Verification items for the finished model (mm, model axes). A direction names the side the tool comes from. Give positions to 0.01 mm unless a question says otherwise; leave off trailing zeros. Order: outer loops, then holes, each group sorted by start corner. A loop starts at its lowest first (then second) coordinate and runs counter-clockwise, first axis right, second up. Notation, with made-up numbers: (70, 63.5) - (113, 63.5) arc R20 cw to (113, 82.5) - close; hole circle Ø1 at (-15.5, 3). An arc over 180 degrees is marked (long way). Answer as a JSON object with one key per item and string values. Group by question number.
(1) Mould release check, pull along Z, two halves, no side actions. Record for faces 6 (the face through (2.465, -7.413, -11.197)), 7 (the face through (2.465, 7.345, -11.241)), 8 (the face through (-3, 0, 10)), 9 (the face through (2.46, 12.85, -3.89)): +Z half, -Z half, draft (parallel to the pull), parting line (faces both ways), or undercut.
(2) Thickness scan on line 1 (Y direction, x = 3.55, z = 0); line 2 (Y direction, x = 4, z = 12.5); line 3 (Y direction, x = -4.25, z = 0). Record the ranges inside material, lowest first.
(3) Section check B-B (y = -9.25). Record the boundary of the cut face in (x, z), then the cut area to 3 significant figures.
(4) Section check A-A (x = -4.5). Record the boundary of the cut face in (y, z), then the cut area to 3 significant figures.
(5) Depth check by flat-ended pin: pin 1 Ø0.9 at (y, z) = (0.5, 5.5) entering from -X; pin 2 Ø1 at (x, y) = (1.5, 9) entering from -Z; pin 3 Ø6 at (x, z) = (-4.5, 11.5) entering from -Y. Enter the tip coordinate at first touch or a pass-through.
(6) Access from +Z, -Z, +X, -X, +Y, -Y to the whole of each face (thin tool, end or side, straight path). Record for faces 1 (the face through (2.46, -0.71, 12.23)), 2 (the face through (2.465, -12.842, 3.814)), 3 (the face through (2.46, 13.4, -0.82)), 4 (the face through (2.465, -10.747, 8.051)), 5 (the face through (2.465, -4.631, -12.605)).
```python
from build123d import *

# Parameters (mm, degrees)
BASPROSKE_W         = 5
BASPROSKE_H         = 14.5
TOOTHCUT_DEPTH      = 22.106870919
TEETHCUTS_COUNT     = 27
TEETHCUTS_ANGLE     = 346.666666667
BORSKE_R            = 1.5
BORE_DEPTH          = 50.0000508
SKETCH2_R           = 10
BOSS_EXTRUDE1_DEPTH = 7
CUT_EXTRUDE3_START  = -7
SKETCH3_R           = 1.5
CUT_EXTRUDE3_DEPTH  = 7


with BuildPart() as part:
    # BasProSke → Base-Revolve (revolve)
    with BuildSketch(Plane(origin=(0, 0, 0), x_dir=(1, 0, 0), z_dir=(0, 1, 0)), mode=Mode.PRIVATE) as base_revolve_sk:
        with Locations((2.5, 7.25)):
            Rectangle(BASPROSKE_W, BASPROSKE_H)
    revolve(base_revolve_sk.sketch.rotate(Axis((-10, 0, 0), (1, 0, 0)), 180), axis=Axis((-10, 0, 0), (1, 0, 0)))

    # TooCutSke → ToothCut (cut, through all)
    with BuildSketch(Plane(origin=(0, 0, 0), x_dir=(0, 0, -1), z_dir=(1, 0, 0))):
        with BuildLine():
            ThreePointArc((0.474054864, 12.239823242), (0, 12.249), (-0.474054864, 12.239823242))
            ThreePointArc((-0.474054864, 12.239823242), (-0.820231692, 13.40120918), (-1.416685779, 14.456149092))
            ThreePointArc((-1.416685779, 14.456149092), (0, 14.5254), (1.416685779, 14.456149092))
            ThreePointArc((1.416685779, 14.456149092), (0.820231692, 13.40120918), (0.474054864, 12.239823242))
        make_face()
    toothcut = extrude(amount=TOOTHCUT_DEPTH, mode=Mode.SUBTRACT)

    # TeethCuts: ToothCut ×27 about axis
    teethcuts_axis = Axis((-10, 0, 0), (1, 0, 0))
    for i in range(1, TEETHCUTS_COUNT):
        add(toothcut.rotate(teethcuts_axis, i * TEETHCUTS_ANGLE / (TEETHCUTS_COUNT - 1)), mode=Mode.SUBTRACT)

    # BorSke → Bore (cut, symmetric)
    with BuildSketch(Plane(origin=(0, 0, 0), x_dir=(0, 0, -1), z_dir=(1, 0, 0))):
        with Locations(Location((0, 0, 0), (0, 0, 180))):
            Circle(BORSKE_R)
    extrude(amount=BORE_DEPTH, both=True, mode=Mode.SUBTRACT)

    # Sketch2 → Boss-Extrude1 (add)
    with BuildSketch(Plane.ZY):
        with Locations(Location((0, 0, 0), (0, 0, 180))):
            Circle(SKETCH2_R)
    extrude(amount=BOSS_EXTRUDE1_DEPTH)

    # Sketch3 → Cut-Extrude3 (cut)
    with BuildSketch(Plane.ZY.offset(7).offset(CUT_EXTRUDE3_START)):
        Circle(SKETCH3_R)
        with Locations((5, 0)):
            Circle(SKETCH3_R)
        with Locations((-5, 0)):
            Circle(SKETCH3_R)
    extrude(amount=CUT_EXTRUDE3_DEPTH, mode=Mode.SUBTRACT)


solid = part.part
```
Solutions:
{
 "1": {"face 6": "-Z half", "face 7": "undercut", "face 8": "parting line", "face 9": "undercut"},
 "2": {"line 1": "y = -14.5 to -1.5, 1.5 to 12.25", "line 2": "y = -6.03 to -4.55, -3.09 to -1.27, -0.2 to 1.65, 2.82 to 4.55, 6.7 to 7.35", "line 3": "y = -10 to -1.5, 1.5 to 10"},
 "3": {"outline": "(-7, -3.8) - (0, -3.8) - (0, -8.91) - (5, -8.91) - (5, 8.91) - (0, 8.91) - (0, 3.8) - (-7, 3.8) - close", "area": "142 mm2"},
 "4": {"outline": "circle Ø20 at (0, 0); hole circle Ø3 at (0, -5); hole circle Ø3 at (0, 0); hole circle Ø3 at (0, 5)", "area": "293 mm2"},
 "5": {"pin 1": "stops at x = 0", "pin 2": "stops at z = -10.66", "pin 3": "stops at y = -5.27"},
 "6": {"face 1": "+Z, +X, -X", "face 2": "+X, -X", "face 3": "+X, -X, +Y", "face 4": "+X, -X, -Y", "face 5": "-Z, +X, -X"}
}
